Verification items for the finished model (mm, model axes). Face numbers are marked on the shaded views. A direction names the side the tool comes from. Give positions to 0.01 mm unless a question says otherwise; leave off trailing zeros. Loops run counter-clockwise (first coordinate to the right, second up) from the corner with the lowest first, then second, coordinate; pieces in that order, holes last. Notation, with made-up numbers: (56.5, -14) - (112.5, -14) arc R30 cw to (112.5, 13) - close; hole circle Ø2 at (1.25, -21.75). An arc over 180 degrees is marked (long way). One line per item, written item: value. Start each with the question number.
1. Sectioned sample at C-C (y = 9.75). Record the cut outline in (x, z) (3 decimals).
2. Sectioned sample at A-A (z = 0). Record the cut outline in (x, y).
3. Scan lines: L1, parallel to Z at x = 25, y = 8.5 (3 decimals); L2, parallel to X at y = 1.75, z = 7.5; L3, parallel to Y at x = 19, z = 47.5. Record each from-to range of solid material in increasing order. Write a range as [from, to].
4. Sectioned sample at D-D (x = 5.5). Record the cut outline in (y, z) (3 decimals), plus the area to 3 significant figures.
5. Sectioned sample at B-B (x = 24.45). Record the cut outline in (y, z) (3 decimals).
6. Access from +Z, -Z, +X, -X, +Y, -Y to the whole of each face (thin tool, end or side, straight path). Record for the marked faces 1 and 2.
7. Gauge pin test, flat ends, axial feed: pin 1 (6 mm diameter, centred on x = 60.038, z = -60.565, fed in from +Y); pin 2 (2 mm diameter, centred on y = 0.5, z = 5, fed in from -X); pin 3 (9 mm diameter, centred on x = -64.45, z = 69.977, fed in from -Y); pin 4 (9 mm diameter, centred on x = 26, z = -68.5, fed in from +Y). Record the tip position at first contact, or that the pin passes through.
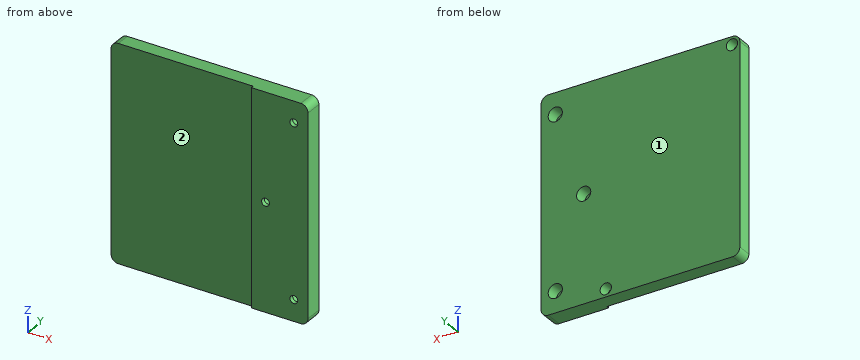
from build123d import *

# Parameters (mm, degrees)
SKETCH1_W           = 140.076
SKETCH1_H           = 151.13
BOSS_EXTRUDE1_DEPTH = 12
SKETCH2_W           = 100.076
SKETCH2_H           = 151.13
CUT_EXTRUDE1_DEPTH  = 2
SKETCH3_R           = 4
CUT_EXTRUDE2_DEPTH  = 8
CUT_EXTRUDE3_REACH  = 105.727
SKETCH4_R           = 2.75
FILLET1_R           = 5.08
SKETCH5_R           = 5
CUT_EXTRUDE4_DEPTH  = 9


with BuildPart() as part:
    # Sketch1 → Boss-Extrude1 (new body)
    with BuildSketch(Plane(origin=(0, 0, 0), x_dir=(1, 0, 0), z_dir=(0, 1, 0))):
        Rectangle(SKETCH1_W, SKETCH1_H)
    extrude(amount=BOSS_EXTRUDE1_DEPTH)

    # Sketch2 → Cut-Extrude1 (cut)
    with BuildSketch(Plane.XZ):
        with Locations((-20, 0)):
            Rectangle(SKETCH2_W, SKETCH2_H)
    extrude(amount=-CUT_EXTRUDE1_DEPTH, mode=Mode.SUBTRACT)

    # Sketch3 → Cut-Extrude2 (cut)
    with BuildSketch(Plane(origin=(0, 12, 0), x_dir=(1, 0, 0), z_dir=(0, 1, 0))):
        with Locations(Location((24.45, 69.977, 0), (0, 0, 270))):
            Circle(SKETCH3_R)
        with Locations(Location((-64.45, -69.977, 0), (0, 0, 270))):
            Circle(SKETCH3_R)
    extrude(amount=-CUT_EXTRUDE2_DEPTH, mode=Mode.SUBTRACT)

    # Sketch4 → Cut-Extrude3 (cut, up to next)
    with BuildSketch(Plane(origin=(0, 12, 0), x_dir=(1, 0, 0), z_dir=(0, 1, 0)), mode=Mode.PRIVATE) as cut_extrude3_sk1:
        with Locations(Location((40.038, 0, 0), (0, 0, 270))):
            Circle(SKETCH4_R)
    cut_extrude3_tool1 = extrude(cut_extrude3_sk1.sketch, amount=-CUT_EXTRUDE3_REACH, mode=Mode.PRIVATE) & part.part
    # Sketch4 → Cut-Extrude3 (cut, up to next)
    with BuildSketch(Plane(origin=(0, 12, 0), x_dir=(1, 0, 0), z_dir=(0, 1, 0)), mode=Mode.PRIVATE) as cut_extrude3_sk2:
        with Locations(Location((60.038, -60.565, 0), (0, 0, 270))):
            Circle(SKETCH4_R)
    cut_extrude3_tool2 = extrude(cut_extrude3_sk2.sketch, amount=-CUT_EXTRUDE3_REACH, mode=Mode.PRIVATE) & part.part
    # Sketch4 → Cut-Extrude3 (cut, up to next)
    with BuildSketch(Plane(origin=(0, 12, 0), x_dir=(1, 0, 0), z_dir=(0, 1, 0)), mode=Mode.PRIVATE) as cut_extrude3_sk3:
        with Locations(Location((60.038, 60.565, 0), (0, 0, 270))):
            Circle(SKETCH4_R)
    cut_extrude3_tool3 = extrude(cut_extrude3_sk3.sketch, amount=-CUT_EXTRUDE3_REACH, mode=Mode.PRIVATE) & part.part
    add(cut_extrude3_tool1.solids().sort_by_distance((40.038, 12, 0))[0], mode=Mode.SUBTRACT)
    add(cut_extrude3_tool2.solids().sort_by_distance((60.038, 12, 60.565))[0], mode=Mode.SUBTRACT)
    add(cut_extrude3_tool3.solids().sort_by_distance((60.038, 12, -60.565))[0], mode=Mode.SUBTRACT)

    # Fillet1
    fillet1_edges = [part.edges().sort_by_distance(p)[0] for p in [
        (70.038, 6, 75.565),
        (-70.038, 7, 75.565),
        (-70.038, 7, -75.565),
        (70.038, 6, -75.565),
    ]]
    fillet(fillet1_edges, radius=FILLET1_R)

    # Sketch5 → Cut-Extrude4 (cut)
    with BuildSketch(Plane(origin=(0, 12, 0), x_dir=(1, 0, 0), z_dir=(0, 1, 0))):
        with Locations(Location((60.038, 60.565, 0), (0, 0, 270))):
            Circle(SKETCH5_R)
        with Locations(Location((40.038, 0, 0), (0, 0, 270))):
            Circle(SKETCH5_R)
        with Locations(Location((60.038, -60.565, 0), (0, 0, 270))):
            Circle(SKETCH5_R)
    extrude(amount=-CUT_EXTRUDE4_DEPTH, mode=Mode.SUBTRACT)


solid = part.part
Results are:
1. outline: (-70.038, -70.485) arc R5.08 ccw to (-64.958, -75.565) - (64.958, -75.565) arc R5.08 ccw to (70.038, -70.485) - (70.038, 70.485) arc R5.08 ccw to (64.958, 75.565) - (-64.958, 75.565) arc R5.08 ccw to (-70.038, 70.485) - close; hole circle Ø8 at (-64.45, 69.977); hole circle Ø8 at (24.45, -69.977); hole circle Ø10 at (40.038, 0); hole circle Ø10 at (60.038, -60.565); hole circle Ø10 at (60.038, 60.565)
2. outline: (-70.04, 2) - (30.04, 2) - (30.04, 0) - (37.29, 0) - (37.29, 3) - (35.04, 3) - (35.04, 12) - (-70.04, 12) - close; (42.79, 0) - (70.04, 0) - (70.04, 12) - (45.04, 12) - (45.04, 3) - (42.79, 3) - close
3. L1: z = [-75.565, -73.939], [-66.015, 75.565]
3. L2: x = [30.04, 70.04]
3. L3: y = [2, 12]
4. outline: (2, -75.565) - (12, -75.565) - (12, 75.565) - (2, 75.565) - close
4. area: 1,510 mm^2
5. outline: (2, -75.565) - (12, -75.565) - (12, -73.977) - (4, -73.977) - (4, -65.977) - (12, -65.977) - (12, 75.565) - (2, 75.565) - close
6. face 1: +Z, -Z, +X, -X, +Y
6. face 2: +Z, -Z, -X, -Y
7. pin 1: stops at y = 3
7. pin 2: stops at x = 30.04
7. pin 3: stops at y = 2
7. pin 4: stops at y = 12
